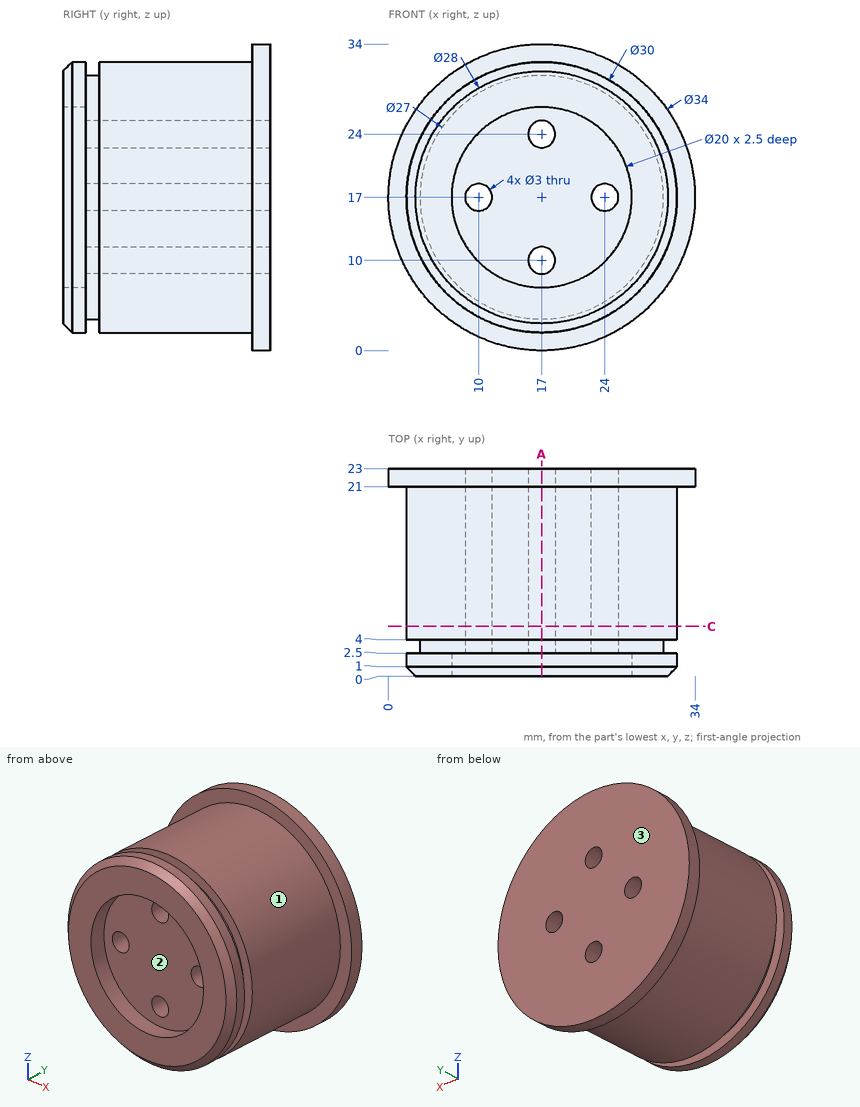
Study the drawing (mm; zero at the part's minimum x, y, z) and answer. Coordinates: 2 decimals unless noted, no trailing zeros. Write each loop counter-clockwise with the first axis right and the second up, starting at its lowest first coordinate (ties: lowest second). Pieces come first, ordered by that corner, then holes. Notation, with made-up numbers: (61.5, 86.25) -> (82.5, 86.25) arc R31 ccw to (82.5, 112.25) -> close; hole circle Ø2 at (-24, 65.5). An arc over 180 degrees is marked (long way). Write each question's results on one line, items separated by ' | '. Start each with the question number.
1) Straight lines are drawn through the part: probe 1 along Z at (x, y) = (16, 12.25); probe 2 along Y at (x, z) = (25.5, 16.5); probe 3 along Z at (x, y) = (10.5, 12.75). For each, find the intervals that lie inside material, in ascending order.
2) A cutting plane is placed at A-A (x = 17). Count the separate pieces of the cut face and the enclosed holes in it, then the cut area to 4 significant figures.
3) A cutting plane is placed at C-C (y = 5.5). Determine the outline of the cut face in (x, z), then the cut area to 3 significant figures.
4) Flat-ended cylindrical pins translate along their axes: pin 1 Ø4 at (x, z) = (17, 10) entering from -Y; pin 2 Ø12 at (y, z) = (6.5, 27.5) entering from -X; pin 3 Ø5 at (y, z) = (20.5, 12) entering from -X; pin 4 Ø2.5 at (x, z) = (24, 17) entering from -Y. Find the tip coordinate at first contact, or state that the pin passes through.
5) For a pull along X with two mould halves and no side action, classify the marked faces 1, 2 and 3 as +X half, -X half, draft (parallel to the pull), parting line (faces both ways), or undercut.
Values follow:
1) probe 1: 2.03 to 8.88, 11.12 to 22.88, 25.12 to 31.97 | probe 2: 2.5 to 23 | probe 3: 3.48 to 15.59, 18.41 to 30.52
2) separate pieces: 3 | enclosed holes: 0 | area: 519.5 mm²
3) outline: circle Ø30 at (17, 17); hole circle Ø3 at (10, 17); hole circle Ø3 at (17, 10); hole circle Ø3 at (17, 24); hole circle Ø3 at (24, 17) | area: 679 mm²
4) pin 1: y = 2.5 | pin 2: x = 2.69 | pin 3: x = 0.19 | pin 4: through
5) face 1: parting line | face 2: undercut | face 3: draft
